Geometry check sheet. Reference: the model listing, model coordinates, mm. Face numbers are marked on the shaded views. A direction names the side the tool comes from. Coordinates: 2 decimals unless noted, no trailing zeros. Loops run counter-clockwise (first coordinate to the right, second up) from the corner with the lowest first, then second, coordinate; pieces in that order, holes last.
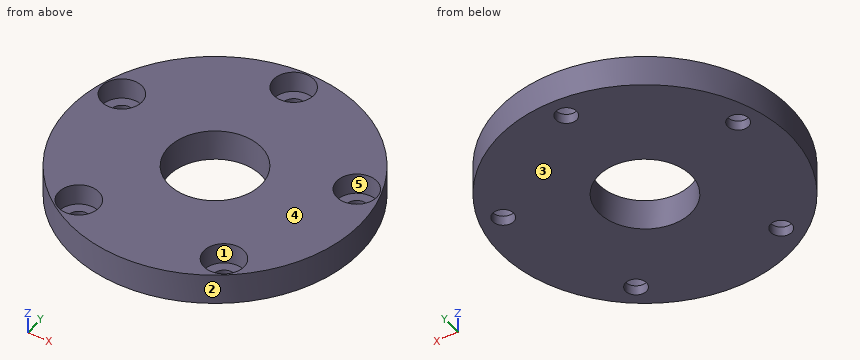
from build123d import *

# Parameters (mm, degrees)
SKETCH1_R               = 23.5
BOSS_EXTRUDE1_DEPTH     = 5
CUT_EXTRUDE1_DEPTH      = 34.608034754
CUT_EXTRUDE1_DEPTH_BACK = 34.608034754
SKETCH5_R               = 7.5
CIRPATTERN1_COUNT       = 5


with BuildPart() as part:
    # Sketch1 → Boss-Extrude1 (new body)
    with BuildSketch(Plane.XY):
        Circle(SKETCH1_R)
    extrude(amount=BOSS_EXTRUDE1_DEPTH)

    # Sketch5 → Cut-Extrude1 (cut, two sides: drawn at the far end of the back side and taken through both)
    with BuildSketch(Plane.XY.offset(5).offset(-CUT_EXTRUDE1_DEPTH_BACK)):
        Circle(SKETCH5_R)
    extrude(amount=CUT_EXTRUDE1_DEPTH + CUT_EXTRUDE1_DEPTH_BACK, mode=Mode.SUBTRACT)

    # Sketch3 → CBORE for M3 Hex Socket Head Cap Screw1 (revolve, cut)
    with BuildSketch(Plane(origin=(0, 20, 5), x_dir=(0, -1, 0), z_dir=(1, 0, 0))):
        Polygon((0, 0), (0, 16.021463052), (1.7, 15), (1.7, 3.4), (3.25, 3.4), (3.25, 0), align=None)
    cbore_for_m3_hex_socket_head_cap_screw1 = revolve(axis=Axis((0, 20, 11.35), (0, 0, -1)), mode=Mode.SUBTRACT)

    # CirPattern1: CBORE for M3 Hex Socket Head Cap Screw1 ×5 about axis
    cirpattern1_axis = Axis((0, 0, 0), (0, 0, 1))
    for i in range(1, CIRPATTERN1_COUNT):
        add(cbore_for_m3_hex_socket_head_cap_screw1.rotate(cirpattern1_axis, i * 360 / CIRPATTERN1_COUNT), mode=Mode.SUBTRACT)


solid = part.part
1) Material ranges on probe 1 along Y at (x, z) = (0, 1.3); probe 2 along X at (y, z) = (-16, 2.55); probe 3 along X at (y, z) = (-18, 4.7), recorded low to high.
Data:
probe 1: y = -23.5 to -7.5, 7.5 to 18.3, 21.7 to 23.5
probe 2: x = -17.21 to -15, -8.51 to 8.51, 15 to 17.21
probe 3: x = -15.11 to -14.45, -9.06 to 9.06, 14.45 to 15.11
2) Section check D-D on z = 4.4. Record the cut outline in (x, y).
Data:
outline: circle Ø47 at (0, 0); hole circle Ø6.5 at (-19.02, 6.18); hole circle Ø6.5 at (-11.76, -16.18); hole circle Ø15 at (0, 0); hole circle Ø6.5 at (0, 20); hole circle Ø6.5 at (11.76, -16.18); hole circle Ø6.5 at (19.02, 6.18)
3) Mould release check, pull along Y, two halves, no side actions. Record for the marked faces 1, 2 and 3: +Y half, -Y half, draft (parallel to the pull), parting line (faces both ways), or undercut.
Data:
face 1: undercut
face 2: parting line
face 3: draft
4) Access from +Z, -Z, +X, -X, +Y, -Y to the whole of each face (thin tool, end or side, straight path). Record for the marked faces 4 and 5.
Data:
face 4: +Z, +X, -X, +Y, -Y
face 5: +Z
5) Section check B-B on x = 0. Record the cut outline in (y, z).
Data:
outline: (-23.5, 0) - (-7.5, 0) - (-7.5, 5) - (-23.5, 5) - close; (7.5, 0) - (18.3, 0) - (18.3, 1.6) - (16.75, 1.6) - (16.75, 5) - (7.5, 5) - close; (21.7, 0) - (23.5, 0) - (23.5, 5) - (23.25, 5) - (23.25, 1.6) - (21.7, 1.6) - close
6) Depth check by flat-ended pin: pin 1 (12 mm diameter, centred on x = 1, y = -14.5, fed in from -Z); pin 2 (1 mm diameter, centred on y = 10.5, z = 2, fed in from -X); pin 3 (2 mm diameter, centred on y = 10.5, z = 0.5, fed in from +X); pin 4 (4 mm diameter, centred on x = 0, y = 20, fed in from +Z). Enter the tip coordinate at first touch or a pass-through.
Data:
pin 1: stops at z = 0
pin 2: stops at x = -21.27
pin 3: stops at x = 21.49
pin 4: stops at z = 1.6
7) Section check A-A on y = 0. Record the cut outline in (x, z), and give its area (3 significant figures).
Data:
outline: (-23.5, 0) - (-7.5, 0) - (-7.5, 5) - (-23.5, 5) - close; (7.5, 0) - (23.5, 0) - (23.5, 5) - (7.5, 5) - close
area: 160 mm2
8) Section check C-C on x = 6. Record the cut outline in (y, z), and give its area (3 significant figures).
Data:
outline: (-22.72, 0) - (-4.5, 0) - (-4.5, 5) - (-22.72, 5) - close; (4.5, 0) - (22.72, 0) - (22.72, 5) - (4.5, 5) - close
area: 182 mm2
